Read the model definition and answer for the solid it produces. Units are mm, in the model's axes. Face numbers are marked on the shaded views. A direction names the side the tool comes from. Coordinates: 2 decimals unless noted, no trailing zeros. Write each loop counter-clockwise with the first axis right and the second up, starting at its lowest first coordinate (ties: lowest second). Pieces come first, ordered by that corner, then holes.
1) The part is cut by section A-A (x = 0). Determine the outline of the cut face in (y, z).
2) Determine the mould class of the marked faces 1, 2 and 3 for opening direction X: +X half, -X half, draft (parallel to the pull), parting line (faces both ways), or undercut.
3) The part is cut by section D-D (x = -9). Determine the outline of the cut face in (y, z), then the cut area to 3 significant figures.
4) Each of these flat-tipped pins is pushed along its axis until it touches: pin 1 Ø6 at (x, y) = (-1.5, -56.5) entering from -Z; pin 2 Ø4 at (y, z) = (-57.5, -14.5) entering from -X; pin 3 Ø10 at (x, y) = (9.5, -62) entering from -Z. Where does it stop, or does it pass through?
5) The part is cut by section B-B (z = 0). Determine the outline of the cut face in (x, y).
6) Find the intervals of material crossed by line 1 (Z direction, x = 0, y = -58.5); line 2 (Y direction, x = 0, z = -16); line 3 (X direction, y = -99, z = -3), in increasing order.
7) Which of the six approach directions +Z, -Z, +X, -X, +Y, -Y give full straight-line access (tool end or side, diameter ignored) to the marked faces 4 and 5?
8) The part is cut by section C-C (y = -51). Determine the outline of the cut face in (x, z).
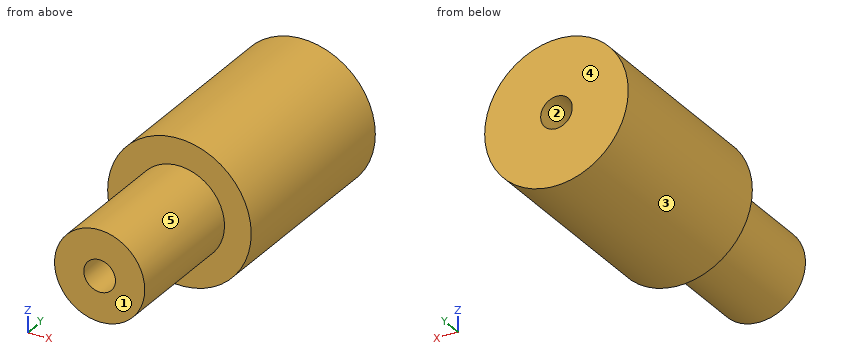
from build123d import *

# Parameters (mm, degrees)
F0_R     = 25
F1_DEPTH = 70
F2_R     = 15.702302
F3_DEPTH = 45
F4_R     = 5.506821
F5_DEPTH = 115.001


with BuildPart() as f1:
    # F0 (on Front) → F1 (new body)
    with BuildSketch(Plane.XZ):
        Circle(F0_R)
    extrude(amount=F1_DEPTH)

    # F2 (on face) → F3 (join)
    with BuildSketch(Plane.XZ.offset(70)):
        Circle(F2_R)
    extrude(amount=F3_DEPTH)

    # F4 (on face) → F5 (cut, through all)
    with BuildSketch(Plane.XZ.offset(115)):
        Circle(F4_R)
        Polygon((-39.301679, 0), (-54.846372, 51.766761), (-54.846372, 0), align=None)
    extrude(amount=-F5_DEPTH, mode=Mode.SUBTRACT)


solid = f1.part
Reported:
1. outline: (-115, -15.7) - (-70, -15.7) - (-70, -25) - (0, -25) - (0, -5.51) - (-115, -5.51) - close; (-115, 5.51) - (0, 5.51) - (0, 25) - (-70, 25) - (-70, 15.7) - (-115, 15.7) - close
2. face 1: draft
2. face 2: undercut
2. face 3: parting line
3. outline: (-115, -12.87) - (-70, -12.87) - (-70, -23.32) - (0, -23.32) - (0, 23.32) - (-70, 23.32) - (-70, 12.87) - (-115, 12.87) - close
3. area: 4,420 mm2
4. pin 1: stops at z = -25
4. pin 2: stops at x = -21.65
4. pin 3: stops at z = -24.59
5. outline: (-25, -70) - (-15.7, -70) - (-15.7, -115) - (-5.51, -115) - (-5.51, 0) - (-25, 0) - close; (5.51, -115) - (15.7, -115) - (15.7, -70) - (25, -70) - (25, 0) - (5.51, 0) - close
6. line 1: z = -25 to -5.51, 5.51 to 25
6. line 2: y = -70 to 0
6. line 3: x = -15.41 to -4.62, 4.62 to 15.41
7. face 4: +Z, -Z, +X, -X, +Y
7. face 5: -Y
8. outline: circle Ø50 at (0, 0); hole circle Ø11.01 at (0, 0)
